```python
from build123d import *

# Parameters (mm, degrees)
BOSS_EXTRUDE1_DEPTH = 49.2125
SKETCH3_R           = 3.175
CUT_EXTRUDE1_DEPTH  = 16.875
SKETCH4_R           = 1.7500092
CUT_EXTRUDE2_DEPTH  = 16.875


with BuildPart() as part:
    # Sketch2 → Boss-Extrude1 (new body, symmetric)
    with BuildSketch(Plane.XY):
        with BuildLine():
            Line((-7.9375, 0), (7.9375, 0))
            Line((7.9375, 0), (7.9375, 15.875))
            Line((7.9375, 15.875), (7.14375, 15.875))
            ThreePointArc((7.14375, 15.875), (6.582483992, 15.642516008), (6.35, 15.08125))
            Line((6.35, 15.08125), (6.35, 2.38125))
            ThreePointArc((6.35, 2.38125), (6.117516008, 1.819983992), (5.55625, 1.5875))
            Line((5.55625, 1.5875), (-7.14375, 1.5875))
            ThreePointArc((-7.14375, 1.5875), (-7.705016008, 1.355016008), (-7.9375, 0.79375))
            Line((-7.9375, 0.79375), (-7.9375, 0))
        make_face()
    extrude(amount=BOSS_EXTRUDE1_DEPTH, both=True)

    # Sketch3 → Cut-Extrude1 (cut, through all)
    with BuildSketch(Plane(origin=(7.9375, 0, 0), x_dir=(0, 0, -1), z_dir=(1, 0, 0))):
        with Locations((-41.275, 7.9375)):
            Circle(SKETCH3_R)
        with Locations((41.275, 7.9375)):
            Circle(SKETCH3_R)
        with Locations((-15.875, 7.9375)):
            Circle(SKETCH3_R)
        with Locations((15.875, 7.9375)):
            Circle(SKETCH3_R)
    extrude(amount=-CUT_EXTRUDE1_DEPTH, mode=Mode.SUBTRACT)

    # Sketch4 → Cut-Extrude2 (cut, through all)
    with BuildSketch(Plane.XZ):
        with Locations((0, -30.1625)):
            Circle(SKETCH4_R)
        with Locations((0, 30.1625)):
            Circle(SKETCH4_R)
    extrude(amount=-CUT_EXTRUDE2_DEPTH, mode=Mode.SUBTRACT)


solid = part.part
```
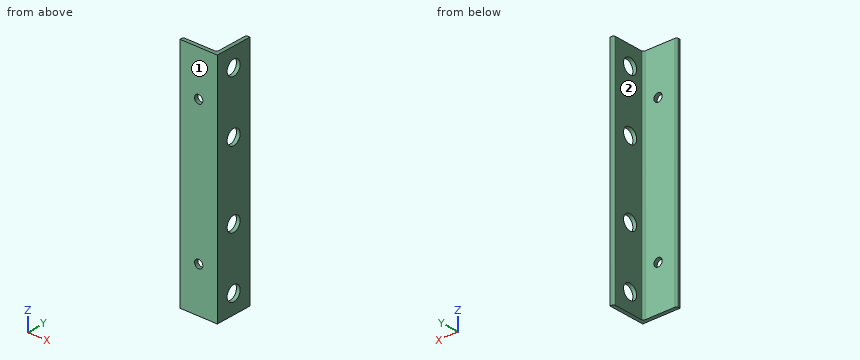
Geometry: final body of the model. Coordinates: model frame, mm. Face numbers are marked on the shaded views. A direction names the side the tool comes from. Round coordinates to 2 decimals unless told otherwise and drop trailing zeros. Order: outer loops, then holes, each group sorted by start corner. A loop starts at its lowest first (then second) coordinate and runs counter-clockwise, first axis right, second up. Notation, with made-up numbers: M 36.25,-2 L 57.25,-2 A27 ccw 57.25,15 Z; hole C 69.25,39.5 d3. An arc over 180 degrees is marked long. Use one line per item in the form item = value. Start each with the question number.
Q1. Cut plane D-D (y = 13). Return loops of the section in (x, z), and give its area (3 significant figures).
Q2. Material intervals for line 1 (Z direction, x = 7, y = 9.25); line 2 (Z direction, x = 0, y = 0.9); line 3 (Y direction, x = 7, z = -41), sorted ascending. Write a range as [from, to].
Q3. Access query for the marked faces 1 and 2. Directions: +Z, -Z, +X, -X, +Y, -Y. A direction counts if a zero-diameter tool reaches every point of the face in a straight line with its end or side. Return the directions, or none.
Q4. Cut plane A-A (x = 0). Return loops of the section in (y, z), and give its area (3 significant figures).
Q5. Pin query (flat end, axial travel): pin 1 Ø6.5 at (x, z) = (-2.5, -0.5) entering from +Y; pin 2 Ø7.5 at (y, z) = (7.94, 15.88) entering from -X; pin 3 Ø4 at (y, z) = (7.94, 41.28) entering from +X. Return the tip coordinate at first contact, or that it passes through.
Geometry results:
q1.outline = M 6.35,-49.21 L 7.94,-49.21 L 7.94,49.21 L 6.35,49.21 Z
q1.area = 156 mm^2
q2.line_1 = [-49.21, -44.17], [-38.38, -18.77], [-12.98, 12.98], [18.77, 38.38], [44.17, 49.21]
q2.line_2 = [-49.21, -31.91], [-28.41, 28.41], [31.91, 49.21]
q2.line_3 = [0, 4.77], [11.1, 15.86]
q3.face_1 = +Z, -Z, +X, -X, -Y
q3.face_2 = +Z, -Z, -X, +Y
q4.outline = M 0,-49.21 L 1.59,-49.21 L 1.59,-31.91 L 0,-31.91 Z; M 0,-28.41 L 1.59,-28.41 L 1.59,28.41 L 0,28.41 Z; M 0,31.91 L 1.59,31.91 L 1.59,49.21 L 0,49.21 Z
q4.area = 145 mm^2
q5.pin_1 = 1.59
q5.pin_2 = 6.35
q5.pin_3 = through
